```python
from build123d import *

# Parameters (mm, degrees)
F1_DEPTH             = 50.8
F2_W                 = 61.9125
F2_H                 = 61.9125
F3_DEPTH             = 57.15
F5_DEPTH             = 50.8
F8_D                 = 6.7564
F8_CSINK_D           = 13.4874
F8_CSINK_ANGLE       = 82
F8_ON_F7_D           = 6.7564
F8_ON_F7_CSINK_D     = 13.4874
F8_ON_F7_CSINK_ANGLE = 82
F9_SIZE              = 6.35
F11_SIZE             = 5.08


# Not quite as in the source:
# - a feature of the source that left no trace in its solid (it failed there, or was rolled back) is left out
# - a feature names something its author has since deleted; it is built from what else it names


with BuildPart() as f1:
    # F0 (on Top) → F1 (new body)
    with BuildSketch(Plane.XY):
        Polygon((-61.9125, 0), (0, 0), (0, 61.9125), (-11.1125, 61.9125), (-11.1125, 11.1125), (-61.9125, 11.1125), align=None)
    extrude(amount=F1_DEPTH)

    # F2 (on Top) → F3 (join)
    with BuildSketch(Plane.XY):
        with Locations((-30.95625, 30.95625)):
            Rectangle(F2_W, F2_H)
    extrude(amount=-F3_DEPTH)

    # F4 (on face) → F5 (join)
    with BuildSketch(Plane(origin=(0, 0, -57.15), x_dir=(1, 0, 0), z_dir=(0, 0, -1))):
        Polygon((0, -61.9125), (0, 0), (-61.9125, 0), (-61.9125, -9.525), (-9.525, -9.525), (-9.525, -61.9125), align=None)
    extrude(amount=F5_DEPTH)

    # F8 (through all)
    with Locations(Plane.YZ):
        with Locations((46.0375, 34.925), (20.6375, 9.525), (20.6375, -66.675), (46.0375, -92.075)):
            CounterSinkHole(F8_D / 2, F8_CSINK_D / 2, counter_sink_angle=F8_CSINK_ANGLE)

    # F8 on F7 (through all)
    with Locations(Plane.XZ):
        with Locations((-20.6375, 34.925), (-46.0375, 9.525), (-46.0375, -66.675), (-20.6375, -92.075)):
            CounterSinkHole(F8_ON_F7_D / 2, F8_ON_F7_CSINK_D / 2, counter_sink_angle=F8_ON_F7_CSINK_ANGLE)

    # F9
    f9_edges = [f1.edges().sort_by_distance(p)[0] for p in [
        (0, 0, -28.575),
    ]]
    chamfer(f9_edges, length=F9_SIZE)

    # F11
    f11_edges = [f1.edges().sort_by_distance(p)[0] for p in [
        (-34.13125, 0, 50.8),
        (-3.175, 3.175, 50.8),
        (0, 34.13125, 50.8),
        (-3.175, 3.175, -107.95),
        (-34.13125, 0, -107.95),
        (0, 34.13125, -107.95),
        (-61.9125, 0, -28.575),
        (0, 61.9125, -28.575),
    ]]
    chamfer(f11_edges, length=F11_SIZE)


solid = f1.part
```
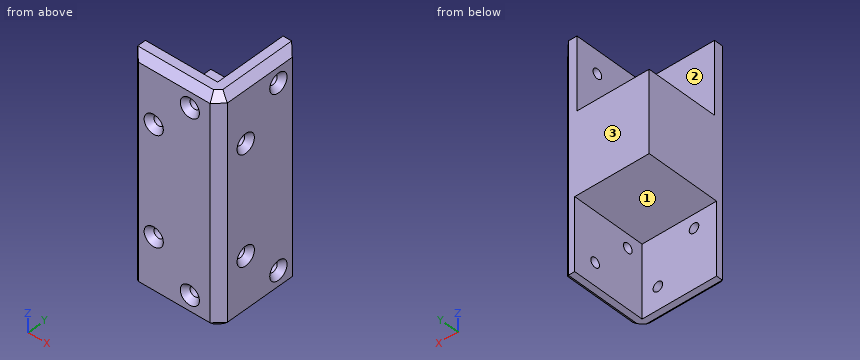
Part model, mm, in its own coordinate system. Face numbers are marked on the shaded views. A direction names the side the tool comes from. Round coordinates to 2 decimals unless told otherwise and drop trailing zeros. Put each result on its own line as item: value. Start each with the question number.
1. Tool access for the marked faces 1, 2 and 3: list every direction of +Z, -Z, +X, -X, +Y, -Y with a clear straight run to the whole face (end or side of a thin tool).
2. Slice it at D-D on y = 22. State how many separate pieces and enclosed holes the cut face has, then the cut area to 3 significant figures.
3. Drill centre lines: probe 1 along Y at (x, z) = (-28, 9); probe 2 along Z at (x, y) = (-45, 42); probe 3 along X at (y, z) = (56, 10.5). Where is each one in solid material? Low to high. Write a range as [from, to].
4. Drop flat-ended pins along their axis: pin 1 (8 mm diameter, centred on x = -46.04, z = 9.52, fed in from -Y); pin 2 (4 mm diameter, centred on x = -20.64, z = 34.92, fed in from +Y); pin 3 (2 mm diameter, centred on y = 40.5, z = -69, fed in from -X) (3 decimals); pin 4 (9 mm diameter, centred on y = 20.64, z = -66.68, fed in from +X). Give the stop position or say it passes through.
Findings:
1. face 1: -Z, -X, +Y
1. face 2: +Z, -X, +Y
1. face 3: +Z, -Z, +X, -X, +Y
2. separate pieces: 3
2. enclosed holes: 0
2. area: 4,410 mm2
3. probe 1: [0, 11.11]
3. probe 2: [-57.15, 0]
3. probe 3: [-11.11, 0]
4. pin 1: y = 3.15
4. pin 2: through
4. pin 3: x = -9.525
4. pin 4: x = -2.57
